Work out the finished part from the listing and answer in its coordinate system (mm). A direction names the side the tool comes from. Give positions to 0.01 mm unless a question says otherwise; leave off trailing zeros. Loops run counter-clockwise (first coordinate to the right, second up) from the corner with the lowest first, then second, coordinate; pieces in that order, holes last.
```python
from build123d import *


with BuildPart() as f1:
    # F0 (on Front) → F1 (revolve)
    with BuildSketch(Plane.XZ):
        Polygon((2.25, -1.5448883603), (2.25, -2.4948883603), (3.7, -2.4948883603), (3.7, -1.4948883603), (3.75, -1.4948883603), (5.2, -1.4948883603), (5.2, 1.4948883603), (3.75, 1.4948883603), (3.7, 1.4948883603), (3.7, 2.4948883603), (2.25, 2.4948883603), (2.25, 1.5448883603), (2.25, 1.4948883603), (2.25, -1.4948883603), align=None)
    revolve(axis=Axis((0, 0, 0), (0, 0, -1)))


with BuildPart() as f1b:
    # F0 (on Front) → F1, piece 2 (revolve)
    with BuildSketch(Plane.XZ):
        Polygon((3.75, -2.4948883603), (6.75, -2.4948883603), (6.75, 2.4948883603), (3.75, 2.4948883603), (3.75, 1.5448883603), (5.25, 1.5448883603), (5.25, -1.5448883603), (3.75, -1.5448883603), align=None)
    revolve(axis=Axis((0, 0, 0), (0, 0, -1)))


solid = f1b.part
```
Q1. Section A-A on x = 0 is taken. Give the vertices of the cut face in (y, z).
Q2. Determine the mould class of faces 3 (the face through (-3.746, -0.165, 2.013)), 4 (the face through (3, 3, 2.495)), 5 (the face through (-1.46, 6.59, 0.03)) for opening direction Y: +Y half, -Y half, draft (parallel to the pull), parting line (faces both ways), or undercut.
Q3. Consider line 1 along Y through (x, z) = (0, 2.3); line 2 along Z through (x, y) = (-4.75, 0.25); line 3 along X through (y, z) = (0, -0.8). Determine where each line is inside the solid, lowest interval first.
Q4. Which of the six approach directions +Z, -Z, +X, -X, +Y, -Y give full straight-line access (tool end or side, diameter ignored) to faces 1 (the face through (-1, -4, -1.545)), 2 (the face through (-3, 3, -2.495))?
Q5. Section C-C on z = 0.6 is taken. Give the vertices of the cut face in (x, y).
Q6. Given pin 1 (1 mm diameter, centred on x = 2.5, z = 1, fed in from +Y); pin 2 (5 mm diameter, centred on x = 2.5, y = 2.5, fed in from +Z); pin 3 (2 mm diameter, centred on x = -4.5, z = -2, fed in from -Y); pin 4 (1.5 mm diameter, centred on y = -1, z = -2, fed in from +X), each flat-ended and moving along its own axis, determine where each tip first touches the part or whether it passes through.
Q7. Section D-D on y = 5 is taken. Give the vertices of the cut face in (x, z).
Check result:
1. outline: (-6.75, -2.49) - (-3.75, -2.49) - (-3.75, -1.54) - (-5.25, -1.54) - (-5.25, 1.54) - (-3.75, 1.54) - (-3.75, 2.49) - (-6.75, 2.49) - close; (3.75, -2.49) - (6.75, -2.49) - (6.75, 2.49) - (3.75, 2.49) - (3.75, 1.54) - (5.25, 1.54) - (5.25, -1.54) - (3.75, -1.54) - close
2. face 3: undercut
2. face 4: draft
2. face 5: parting line
3. line 1: y = -6.75 to -3.75, 3.75 to 6.75
3. line 2: z = -2.49 to -1.54, 1.54 to 2.49
3. line 3: x = -6.75 to -5.25, 5.25 to 6.75
4. face 1: none
4. face 2: -Z, +X, -X, +Y, -Y
5. outline: circle Ø13.5 at (0, 0); hole circle Ø10.5 at (0, 0)
6. pin 1: stops at y = 6.45
6. pin 2: stops at z = 2.49
6. pin 3: stops at y = -5.77
6. pin 4: stops at x = 6.75
7. outline: (-4.53, -2.49) - (4.53, -2.49) - (4.53, 2.49) - (-4.53, 2.49) - close; hole (-1.6, -1.54) - (1.6, -1.54) - (1.6, 1.54) - (-1.6, 1.54) - close
